```python
from build123d import *

# Parameters (mm, degrees)
BOSS_EXTRUDE2_DEPTH = 1
SKETCH2_W           = 0.5
SKETCH2_H           = 0.51
BOSS_EXTRUDE3_DEPTH = 25.69
SKETCH4_W           = 0.5
SKETCH4_H           = 0.51
BOSS_EXTRUDE4_DEPTH = 2.76
SKETCH5_R           = 2.51
BOSS_EXTRUDE5_DEPTH = 7
FILLET2_R           = 2.51


with BuildPart() as part:
    # Sketch1 → Boss-Extrude2 (new body)
    with BuildSketch(Plane.XY):
        with BuildLine():
            Line((-1.731328969, 2.45), (1.731328969, 2.45))
            ThreePointArc((1.731328969, 2.45), (0, -3), (-1.731328969, 2.45))
        make_face()
    extrude(amount=BOSS_EXTRUDE2_DEPTH)

    # Sketch2 → Boss-Extrude3 (add)
    with BuildSketch(Plane(origin=(0, 0, 0), x_dir=(-1, 0, 0), z_dir=(0, 0, -1))):
        with Locations((0, 1.305)):
            Rectangle(SKETCH2_W, SKETCH2_H)
        with Locations((0, -1.525)):
            Rectangle(SKETCH2_W, SKETCH2_H)
    extrude(amount=BOSS_EXTRUDE3_DEPTH)

    # Sketch4 → Boss-Extrude4 (add)
    with BuildSketch(Plane(origin=(0, 0, -25.69), x_dir=(-1, 0, 0), z_dir=(0, 0, -1))):
        with Locations((0, -1.525)):
            Rectangle(SKETCH4_W, SKETCH4_H)
    extrude(amount=BOSS_EXTRUDE4_DEPTH)

    # Sketch5 → Boss-Extrude5 (add)
    with BuildSketch(Plane.XY.offset(1)):
        with Locations((0, -0.09)):
            Circle(SKETCH5_R)
    extrude(amount=BOSS_EXTRUDE5_DEPTH)

    # Fillet2
    fillet2_edges = [part.edges().sort_by_distance(p)[0] for p in [
        (-2.51, -0.09, 8),
    ]]
    fillet(fillet2_edges, radius=FILLET2_R)


solid = part.part
```
Input: part model. Units: mm. Frame: model coordinates. A direction names the side the tool comes from. Round coordinates to 2 decimals unless told otherwise and drop trailing zeros. Write each loop counter-clockwise with the first axis right and the second up, starting at its lowest first coordinate (ties: lowest second). Pieces come first, ordered by that corner, then holes. Notation, with made-up numbers: (78.5, 30) - (121.5, 30) arc R16 ccw to (121.5, 49) - close; hole circle Ø2 at (58, -30). An arc over 180 degrees is marked (long way). Write item = value, one per line.
(1) Section query A-A on z = -17. Output: boundary loops of the cut face in (x, y).
Geometry check:
outline = (-0.25, -1.78) - (0.25, -1.78) - (0.25, -1.27) - (-0.25, -1.27) - close; (-0.25, 1.05) - (0.25, 1.05) - (0.25, 1.56) - (-0.25, 1.56) - close
(2) Contact query for flat-ended pins moving along their axis: pin 1 Ø1 at (x, z) = (-1, -4) entering from -Y; pin 2 Ø0.6 at (x, z) = (0, -10.5) entering from +Y; pin 3 Ø1.5 at (y, z) = (-2, -8) entering from +X; pin 4 Ø3 at (x, z) = (-1.5, 2) entering from -Y. Output: stop coordinate, or through.
Geometry check:
pin_1 = through
pin_2 = 1.56
pin_3 = 0.25
pin_4 = -2.98
(3) Section query D-D on z = 6. Output: boundary loops of the cut face in (x, y).
Geometry check:
outline = circle Ø4.92 at (0, -0.09)
(4) Material intervals for probe 1 along Z at (x, y) = (-2.5, -0.6); probe 2 along X at (y, z) = (-1.4, -20); probe 3 along Y at (x, z) = (-0.8, 4), sorted ascending.
Geometry check:
probe_1 = 0 to 1
probe_2 = -0.25 to 0.25
probe_3 = -2.47 to 2.29
(5) Section query B-B on x = 0.8. Output: boundary loops of the cut face in (y, z).
Geometry check:
outline = (-2.89, 0) - (2.45, 0) - (2.45, 1) - (2.29, 1) - (2.29, 5.49) arc R2.38 ccw to (-2.47, 5.49) - (-2.47, 1) - (-2.89, 1) - close
(6) Access query for faces 1 (the flat face through (0, 2.45, 0.5)), 2 (the cylindrical face through (-0.54, -2.54, 3.21)). Directions: +Z, -Z, +X, -X, +Y, -Y. A direction counts if a zero-diameter tool reaches every point of the face in a straight line with its end or side. Return the directions, or none.
Geometry check:
face_1 = +Z, -Z, +X, -X, +Y
face_2 = +Z
(7) Section query C-C on y = 2.05. Output: boundary loops of the cut face in (x, z), then the cut area to 3 significant figures.
Geometry check:
outline = (-2.19, 0) - (2.19, 0) - (2.19, 1) - (1.31, 1) - (1.31, 5.49) arc R1.31 ccw to (-1.31, 5.49) - (-1.31, 1) - (-2.19, 1) - close
area = 18.9 mm^2
